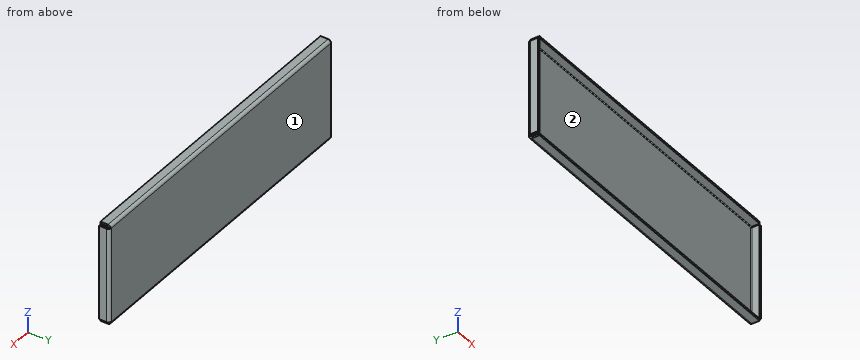
```python
from build123d import *

# Parameters (mm, degrees)
SKETCH1_W                    = 305
SKETCH1_H                    = 10
BASE_FLANGE3_DEPTH           = 2
EDGE_FLANGE1_STRIP_W         = 9.4732
EDGE_FLANGE1_STRIP_H         = 2
EDGE_FLANGE1_STRIP_CUT_DEPTH = 305
EDGE_FLANGE1_DEPTH           = 305
EDGE_FLANGE2_STRIP_W         = 9.4732
EDGE_FLANGE2_STRIP_H         = 2
EDGE_FLANGE2_STRIP_CUT_DEPTH = 305
EDGE_FLANGE2_DEPTH           = 305
EDGE_FLANGE3_STRIP_W         = 9.4732
EDGE_FLANGE3_STRIP_H         = 2
EDGE_FLANGE3_STRIP_CUT_DEPTH = 90.5268
EDGE_FLANGE3_DEPTH           = 90.5268
EDGE_FLANGE4_STRIP_W         = 9.4732
EDGE_FLANGE4_STRIP_H         = 2
EDGE_FLANGE4_STRIP_CUT_DEPTH = 90.5268
EDGE_FLANGE4_DEPTH           = 90.5268


# Sheet-metal steps are written as plain solids
with BuildPart() as part:
    # Sketch1 → Base-Flange3 (new body)
    with BuildSketch(Plane.XY):
        Rectangle(SKETCH1_W, SKETCH1_H)
    extrude(amount=-BASE_FLANGE3_DEPTH)

    # Edge-Flange1 strip (across the edge) → Edge-Flange1 strip cut (cut)
    with BuildSketch(Plane(origin=(-152.5, 5, -2), x_dir=(0, -1, 0), z_dir=(1, 0, 0))):
        with Locations((-2, -1)):
            Rectangle(EDGE_FLANGE1_STRIP_W, EDGE_FLANGE1_STRIP_H)
    extrude(amount=EDGE_FLANGE1_STRIP_CUT_DEPTH, mode=Mode.SUBTRACT)

    # Edge-Flange1 section (across the edge) → Edge-Flange1 (add)
    with BuildSketch(Plane(origin=(-152.5, 5, -2), x_dir=(0, -1, 0), z_dir=(1, 0, 0))):
        with BuildLine():
            Line((0, 0.7366), (0, 94))
            Line((0, 94), (2, 94))
            Line((2, 94), (2, 0.7366))
            ThreePointArc((2, 0.7366), (2.215745145, 0.215745145), (2.7366, 0))
            Line((2.7366, 0), (2.7366, -2))
            ThreePointArc((2.7366, -2), (0.801531583, -1.198468417), (0, 0.7366))
        make_face()
    extrude(amount=EDGE_FLANGE1_DEPTH)

    # Edge-Flange2 strip (across the edge) → Edge-Flange2 strip cut (cut)
    with BuildSketch(Plane(origin=(-152.5, 3, -96), x_dir=(0, 0, 1), z_dir=(1, 0, 0))):
        with Locations((-2, -1)):
            Rectangle(EDGE_FLANGE2_STRIP_W, EDGE_FLANGE2_STRIP_H)
    extrude(amount=EDGE_FLANGE2_STRIP_CUT_DEPTH, mode=Mode.SUBTRACT)

    # Edge-Flange2 section (across the edge) → Edge-Flange2 (add)
    with BuildSketch(Plane(origin=(-152.5, 3, -96), x_dir=(0, 0, 1), z_dir=(1, 0, 0))):
        with BuildLine():
            Line((0, 0.7366), (0, 8))
            Line((0, 8), (2, 8))
            Line((2, 8), (2, 0.7366))
            ThreePointArc((2, 0.7366), (2.215745145, 0.215745145), (2.7366, 0))
            Line((2.7366, 0), (2.7366, -2))
            ThreePointArc((2.7366, -2), (0.801531583, -1.198468417), (0, 0.7366))
        make_face()
    extrude(amount=EDGE_FLANGE2_DEPTH)

    # Edge-Flange3 strip (across the edge) → Edge-Flange3 strip cut (cut)
    with BuildSketch(Plane(origin=(-152.5, 3, -2.7366), x_dir=(1, 0, 0), z_dir=(0, 0, -1))):
        with Locations((-4, -1)):
            Rectangle(EDGE_FLANGE3_STRIP_W, EDGE_FLANGE3_STRIP_H)
    extrude(amount=EDGE_FLANGE3_STRIP_CUT_DEPTH, mode=Mode.SUBTRACT)

    # Edge-Flange3 section (across the edge) → Edge-Flange3 (add)
    with BuildSketch(Plane(origin=(-152.5, 3, -2.7366), x_dir=(1, 0, 0), z_dir=(0, 0, -1))):
        with BuildLine():
            Line((-2, 0.7366), (-2, 8))
            Line((-2, 8), (0, 8))
            Line((0, 8), (0, 0.7366))
            ThreePointArc((0, 0.7366), (0.215745145, 0.215745145), (0.7366, 0))
            Line((0.7366, 0), (0.7366, -2))
            ThreePointArc((0.7366, -2), (-1.198468417, -1.198468417), (-2, 0.7366))
        make_face()
    extrude(amount=EDGE_FLANGE3_DEPTH)

    # Edge-Flange4 strip (across the edge) → Edge-Flange4 strip cut (cut)
    with BuildSketch(Plane(origin=(152.5, 3, -93.2634), x_dir=(-1, 0, 0), z_dir=(0, 0, 1))):
        with Locations((-4, -1)):
            Rectangle(EDGE_FLANGE4_STRIP_W, EDGE_FLANGE4_STRIP_H)
    extrude(amount=EDGE_FLANGE4_STRIP_CUT_DEPTH, mode=Mode.SUBTRACT)

    # Edge-Flange4 section (across the edge) → Edge-Flange4 (add)
    with BuildSketch(Plane(origin=(152.5, 3, -93.2634), x_dir=(-1, 0, 0), z_dir=(0, 0, 1))):
        with BuildLine():
            Line((-2, 0.7366), (-2, 8))
            Line((-2, 8), (0, 8))
            Line((0, 8), (0, 0.7366))
            ThreePointArc((0, 0.7366), (0.215745145, 0.215745145), (0.7366, 0))
            Line((0.7366, 0), (0.7366, -2))
            ThreePointArc((0.7366, -2), (-1.198468417, -1.198468417), (-2, 0.7366))
        make_face()
    extrude(amount=EDGE_FLANGE4_DEPTH)


solid = part.part
```
Work out the finished part from the listing and answer in its coordinate system (mm). Face numbers are marked on the shaded views. Coordinates: 2 decimals unless noted, no trailing zeros. Write each loop counter-clockwise with the first axis right and the second up, starting at its lowest first coordinate (ties: lowest second). Pieces come first, ordered by that corner, then holes.
Q1. A cutting plane is placed at C-C, the plane z = -87. Give the vertices of the cut face in (x, y).
Q2. Determine the mould class of the marked faces 1 and 2 for opening direction Z: released by +Z, released by -Z, zero draft, split by the parting line, or undercut.
Q3. A cutting plane is placed at A-A, the plane y = 0.75. Give the vertices of the cut face in (x, z), then the cut area to 3 significant figures.
Q4. Find the intervals of material crossed by line 1 (X direction, y = 0.75, z = -75); line 2 (Z direction, x = 106, y = -2.5); line 3 (Y direction, x = 75, z = -4.5), in increasing order.
Q5. Each of these flat-tipped pins is pushed along its axis until it touches: pin 1 Ø1 at (x, z) = (-15, -21) entering from -Y; pin 2 Ø0.8 at (y, z) = (0.5, -1.5) entering from +X; pin 3 Ø0.8 at (x, y) = (-153.5, -2) entering from +Z. Where does it stop, or does it pass through?
Q6. A cutting plane is placed at B-B, the plane x = 132.5. Give the vertices of the cut face in (y, z).
Findings below:
1. outline: (-154.5, -5) - (-152.5, -5) - (-152.5, 2.26) arc R0.74 cw to (-151.76, 3) - (151.76, 3) arc R0.74 cw to (152.5, 2.26) - (152.5, -5) - (154.5, -5) - (154.5, 2.26) arc R2.74 ccw to (151.76, 5) - (-151.76, 5) arc R2.74 ccw to (-154.5, 2.26) - close
2. face 1: zero draft
2. face 2: undercut
3. outline: (-154.5, -93.26) - (-152.5, -93.26) - (-152.5, -2.74) - (-154.5, -2.74) - close; (-152.5, -96) - (152.5, -96) - (152.5, -94) - (-152.5, -94) - close; (-152.5, -2) - (152.5, -2) - (152.5, 0) - (-152.5, 0) - close; (152.5, -93.26) - (154.5, -93.26) - (154.5, -2.74) - (152.5, -2.74) - close
3. area: 1,580 mm2
4. line 1: x = -154.5 to -152.5, 152.5 to 154.5
4. line 2: z = -96 to -94, -2 to 0
4. line 3: y = 3 to 5
5. pin 1: stops at y = 3
5. pin 2: stops at x = 152.5
5. pin 3: stops at z = -2.74
6. outline: (-5, -96) - (2.26, -96) arc R2.74 ccw to (5, -93.26) - (5, -2.74) arc R2.74 ccw to (2.26, 0) - (-5, 0) - (-5, -2) - (2.26, -2) arc R0.74 cw to (3, -2.74) - (3, -93.26) arc R0.74 cw to (2.26, -94) - (-5, -94) - close
